```python
from build123d import *

# Parameters (mm, degrees)
SKETCH_W      = 100
SKETCH_H      = 20
PAD_DEPTH     = 3
SKETCH001_W   = 100
SKETCH001_H   = 5
PAD001_DEPTH  = 3
SKETCH002_W   = 100
SKETCH002_H   = 20
SKETCH002_W_2 = 95.5
SKETCH002_H_2 = 3
PAD002_DEPTH  = 3


with BuildPart() as part:
    # Sketch → Pad (new body)
    with BuildSketch(Plane.XY):
        Rectangle(SKETCH_W, SKETCH_H)
    extrude(amount=PAD_DEPTH)

    # Sketch001 (on Face6 of Pad) → Pad001 (join)
    with BuildSketch(Plane.XY.offset(3)):
        with Locations((0, 7.5)):
            Rectangle(SKETCH001_W, SKETCH001_H)
        with Locations((0, -7.5)):
            Rectangle(SKETCH001_W, SKETCH001_H)
    extrude(amount=PAD001_DEPTH)

    # Sketch002 (on Face12 of Pad001) → Pad002 (join)
    with BuildSketch(Plane.XY.offset(6)):
        Rectangle(SKETCH002_W, SKETCH002_H)
        Rectangle(SKETCH002_W_2, SKETCH002_H_2, mode=Mode.SUBTRACT)
    extrude(amount=PAD002_DEPTH)


solid = part.part
```
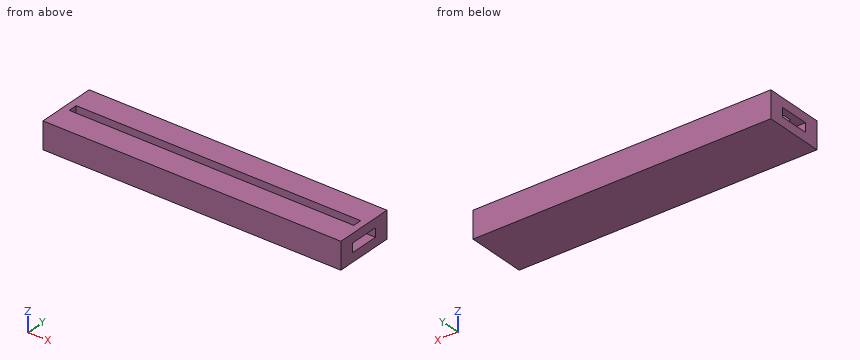
Input: part model. Units: mm. Frame: model coordinates. Give positions to 0.01 mm unless a question says otherwise; leave off trailing zeros. Write each loop counter-clockwise with the first axis right and the second up, starting at its lowest first coordinate (ties: lowest second). Pieces come first, ordered by that corner, then holes. Notation, with made-up numbers: (57, -28.5) - (87, -28.5) arc R32 ccw to (87, 2.5) - close; hole circle Ø6 at (15, -2). An arc over 180 degrees is marked (long way). Write item = value, one per line. Start each with the question number.
1) Material intervals for L1, parallel to Y at x = 45, z = 7; L2, parallel to Z at x = -32.5, y = 1.75; L3, parallel to Y at x = 27.5, z = 3.5, sorted ascending. Write a range as [from, to].
2) Cut plane B-B (y = 3.5). Return loops of the section in (x, z), and give its area (3 significant figures).
3) Cut plane A-A (z = 8). Return loops of the section in (x, y).
4) Cut plane C-C (x = 40.5). Return loops of the section in (y, z).
Answers follow:
q1.L1 = [-10, -1.5], [1.5, 10]
q1.L2 = [0, 3], [6, 9]
q1.L3 = [-10, -5], [5, 10]
q2.outline = (-50, 0) - (50, 0) - (50, 3) - (-50, 3) - close; (-50, 6) - (50, 6) - (50, 9) - (-50, 9) - close
q2.area = 600 mm^2
q3.outline = (-50, -10) - (50, -10) - (50, 10) - (-50, 10) - close; hole (-47.75, -1.5) - (47.75, -1.5) - (47.75, 1.5) - (-47.75, 1.5) - close
q4.outline = (-10, 0) - (10, 0) - (10, 9) - (1.5, 9) - (1.5, 6) - (5, 6) - (5, 3) - (-5, 3) - (-5, 6) - (-1.5, 6) - (-1.5, 9) - (-10, 9) - close
